The model under review builds one solid part; all positions refer to its coordinate system, in mm. Face numbers are marked on the shaded views. A direction names the side the tool comes from. Give positions to 0.01 mm unless a question says otherwise; leave off trailing zeros. Order: outer loops, then holes, each group sorted by start corner. A loop starts at its lowest first (then second) coordinate and runs counter-clockwise, first axis right, second up. Notation, with made-up numbers: (65, 24.5) -> (113, 24.5) arc R31 cw to (113, 52.5) -> close; hole circle Ø10 at (-32, -34.5). An arc over 180 degrees is marked (long way). Use one line per item in the form item = value.
```python
from build123d import *

# Parameters (mm, degrees)
F0_W     = 80
F0_H     = 24
F0_R     = 2.5
F1_DEPTH = 3
F3_DEPTH = 10


with BuildPart() as f1:
    # F0 (on Front) → F1 (new body)
    with BuildSketch(Plane.XZ):
        with Locations((-6.643935, 1.315546)):
            Rectangle(F0_W, F0_H)
        with Locations((-41.943935, -5.634454)):
            Circle(F0_R, mode=Mode.SUBTRACT)
        with Locations((28.656065, -5.634454)):
            Circle(F0_R, mode=Mode.SUBTRACT)
        with Locations((-41.943935, 8.265546)):
            Circle(F0_R, mode=Mode.SUBTRACT)
        with Locations((28.656065, 8.265546)):
            Circle(F0_R, mode=Mode.SUBTRACT)
    extrude(amount=F1_DEPTH)

    # F2 (on face) → F3 (join)
    with BuildSketch(Plane.XY.offset(13.315546)):
        with BuildLine():
            ThreePointArc((18.856003, -29.321047), (-6.757583, -54.764478), (-32.143362, -29.093751))
            Line((-32.143362, -29.093751), (-32.143362, -3))
            Line((-32.143362, -3), (-34.143362, -3))
            Line((-34.143362, -3), (-34.143362, -29.087173))
            ThreePointArc((-34.143362, -29.087173), (-6.761956, -56.764478), (20.856003, -29.323214))
            Line((20.856003, -29.323214), (20.856003, -3))
            Line((20.856003, -3), (18.856003, -3))
            Line((18.856003, -3), (18.856003, -29.321047))
        make_face()
    extrude(amount=-F3_DEPTH)


solid = f1.part
```
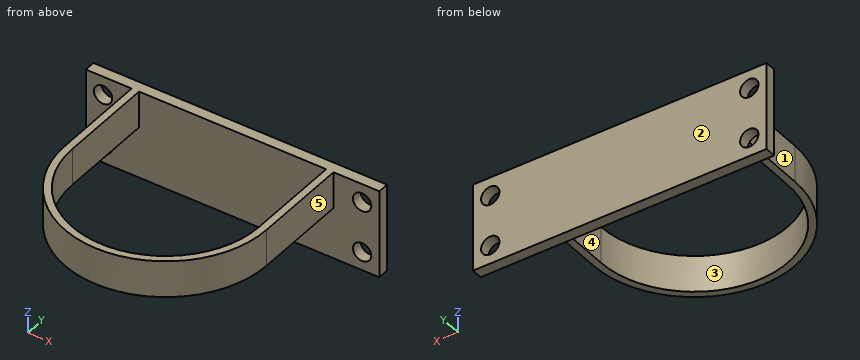
1. Add section A-A on y = -28. Give the boundary of the cut face in (x, z).
Values:
outline = (-34.14, 3.32) -> (-32.14, 3.32) -> (-32.14, 13.32) -> (-34.14, 13.32) -> close; (18.86, 3.32) -> (20.86, 3.32) -> (20.86, 13.32) -> (18.86, 13.32) -> close
2. Add section B-B on x = 7. Give the boundary of the cut face in (y, z), then the cut area to 3 significant figures.
Values:
outline = (-53.14, 3.32) -> (-50.81, 3.32) -> (-50.81, 13.32) -> (-53.14, 13.32) -> close; (-3, -10.68) -> (0, -10.68) -> (0, 13.32) -> (-3, 13.32) -> close
area = 95.3 mm^2
3. Tool access review of the marked faces 4 and 5: name each direction out of +Z, -Z, +X, -X, +Y, -Y from which nothing blocks a thin tool from reaching the whole face with its end or side.
Values:
face_4 = +Z, -Z
face_5 = +Z, -Z, +X, -Y
4. For L1, parallel to X at y = -26, z = 11.5; L2, parallel to Y at x = -4.5, z = -2; L3, parallel to Y at x = -21.5, z = 10.75, list the stretches that pass through material, from the lowest coordinate up.
Values:
L1 = -34.14 to -32.14, 18.86 to 20.86
L2 = -3 to 0
L3 = -52.41 to -49.99, -3 to 0
5. The part is to be moulded in two halves that separate along Y. For the marked faces 1, 2 and 3, say which applies: +Y half, -Y half, draft (parallel to the pull), parting line (faces both ways), or undercut.
Values:
face_1 = draft
face_2 = +Y half
face_3 = undercut
6. Add section D-D on x = -35.5. Give the boundary of the cut face in (y, z).
Values:
outline = (-3, -10.68) -> (0, -10.68) -> (0, 13.32) -> (-3, 13.32) -> close
7. For pin 1 Ø4 at (x, z) = (7, -2) entering from -Y; pin 2 Ø11 at (y, z) = (-18.5, 9.5) entering from +X; pin 3 Ø5 at (x, z) = (-33, 3.5) entering from -Y; pin 4 Ø4.5 at (x, z) = (-41.94, -5.63) entering from -Y, all flat-tipped, find the tip position at first contact; note any pin that passes through.
Values:
pin_1 = -3
pin_2 = 20.86
pin_3 = -42.94
pin_4 = through
8. Add section C-C on z = 1.75. Give the boundary of the cut face in (x, y).
Values:
outline = (-46.64, -3) -> (33.36, -3) -> (33.36, 0) -> (-46.64, 0) -> close
